Design review of the part built by this model. Coordinates are the model's own, in mm. A direction names the side the tool comes from. Coordinates: 2 decimals unless noted, no trailing zeros. Write each loop counter-clockwise with the first axis right and the second up, starting at its lowest first coordinate (ties: lowest second). Pieces come first, ordered by that corner, then holes.
Q1. Machinability: for faces 1 (the flat face through (-7.62, 9, 5)), 2 (the cylindrical face through (-4.866, 1.59, 4.696)), which of the approach directions +Z, -Z, +X, -X, +Y, -Y give a long, thin tool a straight path to every point of the face, cutting with its end or side? Answer none if there is none.
Q2. Mouldability with a two-part tool opening along Y and no side actions: class faces 3 (the flat face through (-6.472, -1.73, 4.696)), 4 (the cylindrical face through (-3.596, 1.404, 4.696)), 5 (the flat face through (-5.08, 9, 5)) as pulls with the +Y half, pulls with the -Y half, needs draft (parallel to the pull), parting line crosses it, or undercut.
Q3. Take a section at C-C (x = 1.5). Give the boundary of the cut face in (y, z) (1 decimal), and give its area (3 significant figures).
Q4. Take a section at A-A (x = -3). Give the boundary of the cut face in (y, z) (3 decimals).
Q5. Take a section at D-D (y = 10.25). Give the boundary of the cut face in (x, z) (3 decimals).
Q6. Insertion check: pin 1 (1.5 mm diameter, centred on x = -5.5, y = 0, fed in from -Z); pin 2 (3 mm diameter, centred on y = 7, z = 5.5, fed in from +X); pin 3 (1.5 mm diameter, centred on x = 0, z = 7, fed in from +Y); pin 4 (1 mm diameter, centred on x = -0.5, y = 4, fed in from +Z) (1 decimal). Each pin has a flat end and moves straight along its axis. Give the tip position at first contact, or say it passes through.
Q7. Take a section at B-B (z = 6). Give the boundary of the cut face in (x, y) (3 decimals).
Q8. For probe 1 along X at (y, z) = (3.5, 2.5); probe 2 along X at (y, z) = (-3, 2.25); probe 3 along X at (y, z) = (7, 5.25), list the stretches that pass through material, from the lowest coordinate up.
```python
from build123d import *

# Parameters (mm, degrees)
F1_DEPTH = 9.525


with BuildPart() as f1:
    # F0 (on Top) → F1 (new body)
    with BuildSketch(Plane.XY):
        with BuildLine():
            Line((-7.62, 0), (-5.291667, -3.510095))
            ThreePointArc((-5.291667, -3.510095), (5.595159, -3.002782), (0, 6.35))
            ThreePointArc((0, 6.35), (-4.86723, 1.48277), (0, -3.384459))
            ThreePointArc((0, -3.384459), (0.635, -2.749459), (0, -2.114459))
            ThreePointArc((0, -2.114459), (-3.59723, 1.48277), (0, 5.08))
            ThreePointArc((0, 5.08), (3.592102, -3.592102), (-5.08, 0))
            Line((-5.08, 0), (-5.08, 17.830187))
            ThreePointArc((-5.08, 17.830187), (-6.35, 19.100187), (-7.62, 17.830187))
            Line((-7.62, 17.830187), (-7.62, 0))
        make_face()
    extrude(amount=F1_DEPTH)


solid = f1.part
```
Response:
1. face 1: +Z, -Z, -X, +Y, -Y
1. face 2: +Z, -Z
2. face 3: pulls with the -Y half
2. face 4: undercut
2. face 5: needs draft
3. outline: (-6.2, 0) - (-4.9, 0) - (-4.9, 9.5) - (-6.2, 9.5) - close; (4.9, 0) - (6.2, 0) - (6.2, 9.5) - (4.9, 9.5) - close
3. area: 25.1 mm2
4. outline: (-5.597, 0) - (-4.1, 0) - (-4.1, 9.525) - (-5.597, 9.525) - close; (-2.35, 0) - (-0.502, 0) - (-0.502, 9.525) - (-2.35, 9.525) - close; (3.468, 0) - (5.316, 0) - (5.316, 9.525) - (3.468, 9.525) - close
5. outline: (-7.62, 0) - (-5.08, 0) - (-5.08, 9.525) - (-7.62, 9.525) - close
6. pin 1: stops at z = 0
6. pin 2: stops at x = 3.17
6. pin 3: stops at y = 6.35
6. pin 4: passes through
7. outline: (-7.62, 0) - (-5.292, -3.51) arc R6.35 ccw (long way) to (0, 6.35) arc R4.867 ccw to (0, -3.384) arc R0.635 ccw to (0, -2.114) arc R3.597 cw to (0, 5.08) arc R5.08 cw (long way) to (-5.08, 0) - (-5.08, 17.83) arc R1.27 ccw to (-7.62, 17.83) - close
8. probe 1: x = -7.62 to -5.08, -4.43 to -2.98, 3.68 to 5.3
8. probe 2: x = -5.63 to -4.1, -1.9 to 0.58, 4.1 to 5.6
8. probe 3: x = -7.62 to -5.08
